Here's how the part is built. I have some questions about the finished solid (model axes, mm). Face numbers are marked on the shaded views. A direction names the side the tool comes from. Round coordinates to 2 decimals unless told otherwise and drop trailing zeros. Write each loop counter-clockwise with the first axis right and the second up, starting at its lowest first coordinate (ties: lowest second). Pieces come first, ordered by that corner, then holes. Notation, with made-up numbers: (-11, -28) -> (45, -28) arc R24 cw to (45, 11) -> close; hole circle Ø4 at (-28.75, 74). An arc over 180 degrees is marked (long way). Put each result on its own line as item: value. Start each with the question number.
1. Suppose I cut it at B-B (x = -15). Please give me the cut outline in (y, z).
2. For pin 1 (12 mm diameter, centred on y = 5, z = 148, fed in from -X); pin 2 (6 mm diameter, centred on x = -4.5, y = 8, fed in from -Z); pin 3 (1 mm diameter, centred on x = -3.5, z = 19.5, fed in from +Y); pin 4 (1.5 mm diameter, centred on x = 13.5, y = -6.5, fed in from +Z), each with a flat end and sliding along its axis, tell me the tip position at first contact or that it passes through.
3. Which directions (+Z, -Z, +X, -X, +Y, -Y) give clear straight access to the entire face, cutting with the end or side of a thin tool? Please do the marked faces 1, 2 and 3.
4. We'd pull the mould along Z, two halves only. Please class the marked faces 4, 5 and 6: +Z half, -Z half, draft (parallel to the pull), parting line (faces both ways), or undercut.
5. Suppose I cut it at A-A (y = 0). Please give me the cut outline in (x, z).
6. Suppose I cut it at D-D (y = 17.5). Please give me the cut outline in (x, z), then the cut area to 3 significant figures.
7. I need wall thicknesses on probe 1 along Z at (x, y) = (-6.5, 9); probe 2 along X at (y, z) = (-9, 22). Which ranges of each line are inside material? Lowest first, please. Write a range as from..to.
```python
from build123d import *

# Parameters (mm, degrees)
SKETCH1_R           = 10.16
BOSS_EXTRUDE1_DEPTH = 177.8
BOSS_EXTRUDE2_START = -12.7
SKETCH2_R           = 19.05
BOSS_EXTRUDE2_DEPTH = 5.08
BOSS_EXTRUDE3_START = -93.98
SKETCH3_R           = 19.05
BOSS_EXTRUDE3_DEPTH = 5.08


with BuildPart() as part:
    # Sketch1 → Boss-Extrude1 (new body)
    with BuildSketch(Plane.XY):
        Circle(SKETCH1_R)
    extrude(amount=BOSS_EXTRUDE1_DEPTH)

    # Sketch2 → Boss-Extrude2 (add)
    with BuildSketch(Plane.XY.offset(177.8).offset(BOSS_EXTRUDE2_START)):
        Circle(SKETCH2_R)
    extrude(amount=BOSS_EXTRUDE2_DEPTH)

    # Sketch3 → Boss-Extrude3 (add)
    with BuildSketch(Plane.XY.offset(177.8).offset(BOSS_EXTRUDE3_START)):
        Circle(SKETCH3_R)
    extrude(amount=BOSS_EXTRUDE3_DEPTH)


solid = part.part
```
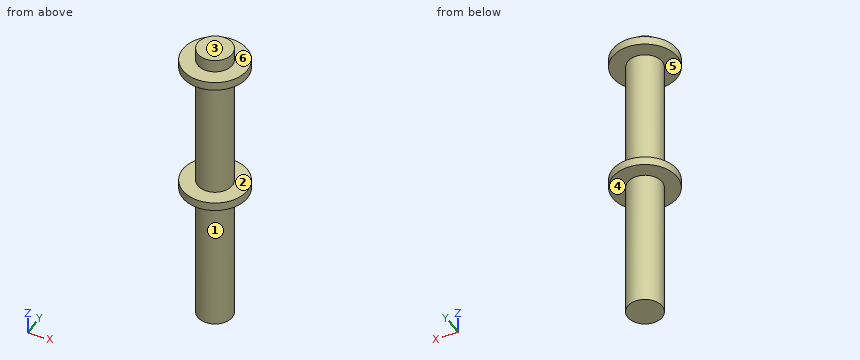
Verdict:
1. outline: (-11.74, 83.82) -> (11.74, 83.82) -> (11.74, 88.9) -> (-11.74, 88.9) -> close; (-11.74, 165.1) -> (11.74, 165.1) -> (11.74, 170.18) -> (-11.74, 170.18) -> close
2. pin 1: stops at x = -10.16
2. pin 2: stops at z = 0
2. pin 3: stops at y = 9.71
2. pin 4: stops at z = 170.18
3. face 1: -Z
3. face 2: none
3. face 3: +Z, +X, -X, +Y, -Y
4. face 4: -Z half
4. face 5: undercut
4. face 6: +Z half
5. outline: (-19.05, 83.82) -> (-10.16, 83.82) -> (-10.16, 0) -> (10.16, 0) -> (10.16, 83.82) -> (19.05, 83.82) -> (19.05, 88.9) -> (10.16, 88.9) -> (10.16, 165.1) -> (19.05, 165.1) -> (19.05, 170.18) -> (10.16, 170.18) -> (10.16, 177.8) -> (-10.16, 177.8) -> (-10.16, 170.18) -> (-19.05, 170.18) -> (-19.05, 165.1) -> (-10.16, 165.1) -> (-10.16, 88.9) -> (-19.05, 88.9) -> close
6. outline: (-7.53, 83.82) -> (7.53, 83.82) -> (7.53, 88.9) -> (-7.53, 88.9) -> close; (-7.53, 165.1) -> (7.53, 165.1) -> (7.53, 170.18) -> (-7.53, 170.18) -> close
6. area: 153 mm^2
7. probe 1: z = 83.82..88.9, 165.1..170.18
7. probe 2: x = -4.71..4.71
